Input: part model. Units: mm. Frame: model coordinates. Face numbers are marked on the shaded views. A direction names the side the tool comes from. Coordinates: 2 decimals unless noted, no trailing zeros. Order: outer loops, then holes, each group sorted by start corner. A loop starts at its lowest first (then second) coordinate and runs counter-clockwise, first axis right, second up.
from build123d import *

# Parameters (mm, degrees)
F0_W     = 23.9
F0_H     = 23
F1_DEPTH = 7
F0_R     = 2.25
F2_DEPTH = 1
F3_W     = 12
F3_H     = 6
F4_DEPTH = 25
F5_R     = 21.25
F6_DEPTH = 10
F0_R_2   = 1.65
F7_DEPTH = 12
F0_R_3   = 1.5
F8_DEPTH = 5


# Not quite as in the source:
# - a feature names something its author has since deleted; it is built from what else it names


with BuildPart() as f1:
    # F0 (on Top) → F1 (new body)
    with BuildSketch(Plane.XY):
        with BuildLine():
            ThreePointArc((2.3312262639, -21.8761373214), (16.3598132295, -14.70906221), (22, 0))
            ThreePointArc((22, 0), (16.3897820024, 14.6756616857), (2.4204503716, 21.86644507))
            ThreePointArc((2.4204503716, 21.86644507), (-0.0200709954, 21.9999908444), (-2.4603446274, 21.8619922311))
            ThreePointArc((-2.4603446274, 21.8619922311), (-21.9999200002, -0.059329476), (-2.3423946746, -21.8749442785))
            ThreePointArc((-2.3423946746, -21.8749442785), (-0.0056159761, -21.9999992832), (2.3312262639, -21.8761373214))
        make_face()
        Rectangle(F0_W, F0_H, mode=Mode.SUBTRACT)
    extrude(amount=-F1_DEPTH)

    # F0 (on Top) → F2 (join)
    with BuildSketch(Plane.XY):
        Rectangle(F0_W, F0_H)
        with Locations((8.75, -8.3)):
            Circle(F0_R, mode=Mode.SUBTRACT)
        with Locations((-3.85, 9.2)):
            Circle(F0_R, mode=Mode.SUBTRACT)
    extrude(amount=-F2_DEPTH)

    # F3 (on face) → F4 (cut)
    with BuildSketch(Plane.YZ.offset(-11.95)):
        with Locations((0, -4.8)):
            Rectangle(F3_W, F3_H)
    extrude(amount=-F4_DEPTH, mode=Mode.SUBTRACT)

    # F5 (on face) → F6 (cut)
    with BuildSketch(Plane(origin=(0, 0, -1), x_dir=(1, 0, 0), z_dir=(0, 0, -1))):
        Circle(F5_R)
    extrude(amount=F6_DEPTH, mode=Mode.SUBTRACT)

    # F0 (on Top) → F7 (join)
    with BuildSketch(Plane.XY):
        with Locations((-3.85, 9.2)):
            Circle(F0_R)
        with Locations((-3.85, 9.2)):
            Circle(F0_R_2, mode=Mode.SUBTRACT)
        with Locations((8.75, -8.3)):
            Circle(F0_R)
        with Locations((8.75, -8.3)):
            Circle(F0_R_2, mode=Mode.SUBTRACT)
    extrude(amount=-F7_DEPTH)

    # F0 (on Top) → F8 (join)
    with BuildSketch(Plane.XY):
        with BuildLine():
            ThreePointArc((-2.4603446274, 21.8619922311), (-0.0200709954, 21.9999908444), (2.4204503716, 21.86644507))
            Line((2.4204503716, 21.86644507), (2.4204503716, 27.4773144078))
            Line((2.4204503716, 27.4773144078), (-2.4603446274, 27.4773144078))
            Line((-2.4603446274, 27.4773144078), (-2.4603446274, 21.8619922311))
        make_face()
        with Locations((0, 24.8148497194)):
            Circle(F0_R_3, mode=Mode.SUBTRACT)
        with BuildLine():
            Line((2.3312262639, -27.183307051), (2.3312262639, -21.8761373214))
            ThreePointArc((2.3312262639, -21.8761373214), (-0.0056159761, -21.9999992832), (-2.3423946746, -21.8749442785))
            Line((-2.3423946746, -21.8749442785), (-2.3423946746, -27.183307051))
            Line((-2.3423946746, -27.183307051), (2.3312262639, -27.183307051))
        make_face()
        with Locations((0, -24.6492363513)):
            Circle(F0_R_3, mode=Mode.SUBTRACT)
    extrude(amount=-F8_DEPTH)


solid = f1.part
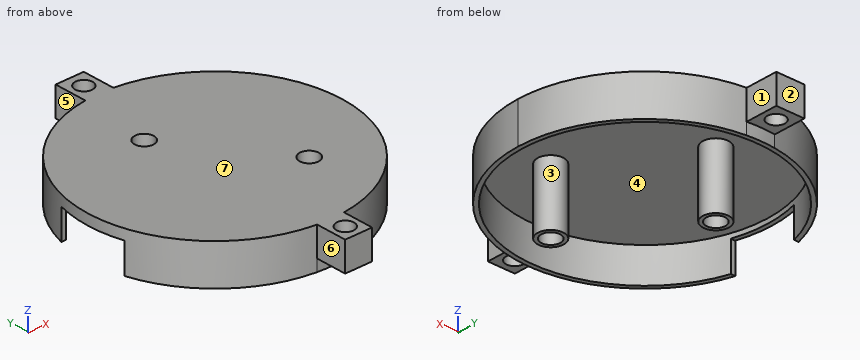
Item 1: Cut plane B-B on z = -8.5. Return loops of the section in (x, y), then the cut area to 3 significant figures.
Response values:
outline: circle Ø4.5 at (-3.85, 9.2); circle Ø4.5 at (8.75, -8.3); hole circle Ø3.3 at (-3.85, 9.2); hole circle Ø3.3 at (8.75, -8.3)
area: 14.7 mm2
Item 2: Ray query, probe 1 along Y at (x, z) = (0, -5.1); probe 2 along Y at (x, z) = (7, -5.5); probe 3 along X at (y, z) = (9, -9.25). Return the intervals inside material, ascending.
Response values:
probe 1: y = -22 to -21.25, 21.25 to 22
probe 2: y = -20.86 to -20.06, -9.71 to -6.89, 20.06 to 20.86
probe 3: x = -6.09 to -5.49, -2.21 to -1.61
Item 3: Access query for the marked faces 4, 5, 6 and 7. Directions: +Z, -Z, +X, -X, +Y, -Y. A direction counts if a zero-diameter tool reaches every point of the face in a straight line with its end or side. Return the directions, or none.
Response values:
face 4: -Z
face 5: +Z, -Z, -X, +Y
face 6: +Z, -Z, -X, -Y
face 7: +Z, +X, -X, +Y, -Y
Item 4: Draft query along X for the marked faces 1, 2 and 3. Return one class per face: pulls with the +X half, pulls with the -X half, needs draft (parallel to the pull), parting line crosses it, or undercut.
Response values:
face 1: pulls with the +X half
face 2: needs draft
face 3: undercut
Item 5: Cut plane A-A on x = 0. Return loops of the section in (y, z), then the cut area to 3 significant figures.
Response values:
outline: (-27.18, -5) - (-26.15, -5) - (-26.15, 0) - (-27.18, 0) - close; (-23.15, -5) - (-22, -5) - (-22, -7) - (-21.25, -7) - (-21.25, -1) - (21.25, -1) - (21.25, -7) - (22, -7) - (22, -5) - (23.31, -5) - (23.31, 0) - (-23.15, 0) - close; (26.31, -5) - (27.48, -5) - (27.48, 0) - (26.31, 0) - close
area: 76.3 mm2
Item 6: Pin query (flat end, axial travel): pin 1 Ø1.3 at (x, y) = (-21, 0.5) entering from -Z; pin 2 Ø5.5 at (x, y) = (0.5, 25) entering from -Z; pin 3 Ø2 at (y, z) = (5.5, -7) entering from +X; pin 4 Ø3 at (x, y) = (-3.85, 9.2) entering from -Z. Return the tip coordinate at first contact, or that it passes through.
Response values:
pin 1: stops at z = -1.8
pin 2: stops at z = -5
pin 3: stops at x = 21.53
pin 4: passes through
Item 7: Cut plane D-D on y = 9.2. Return loops of the section in (x, z), then the cut area to 3 significant figures.
Response values:
outline: (-19.98, -7) - (-19.16, -7) - (-19.16, -1) - (-6.1, -1) - (-6.1, -12) - (-5.5, -12) - (-5.5, 0) - (-19.98, 0) - close; (-2.2, -12) - (-1.6, -12) - (-1.6, -1) - (19.16, -1) - (19.16, -7) - (19.98, -7) - (19.98, 0) - (-2.2, 0) - close
area: 59.8 mm2
Item 8: Cut plane C-C on z = -3. Return loops of the section in (x, y), then the cut area to 3 significant figures.
Response values:
outline: (-21.17, -6) arc R22 ccw to (-2.34, -21.87) - (-2.34, -27.18) - (2.33, -27.18) - (2.33, -21.88) arc R22 ccw to (2.42, 21.87) - (2.42, 27.48) - (-2.46, 27.48) - (-2.46, 21.86) arc R22 ccw to (-21.17, 6) - (-20.39, 6) arc R21.25 cw (long way) to (-20.39, -6) - close; circle Ø4.5 at (-3.85, 9.2); circle Ø4.5 at (8.75, -8.3); hole circle Ø3.3 at (-3.85, 9.2); hole circle Ø3 at (0, -24.65); hole circle Ø3 at (0, 24.81); hole circle Ø3.3 at (8.75, -8.3)
area: 145 mm2
